The model under review builds one solid part; all positions refer to its coordinate system, in mm. Face numbers are marked on the shaded views. A direction names the side the tool comes from. Round coordinates to 2 decimals unless told otherwise and drop trailing zeros. Order: outer loops, then holes, each group sorted by start corner. A loop starts at its lowest first (then second) coordinate and runs counter-clockwise, first axis right, second up. Notation, with made-up numbers: M 85.25,-1 L 144.25,-1 A24 ccw 144.25,25 Z; hole C 32.5,52.25 d3. An arc over 180 degrees is marked long. Answer as a JSON object with one key per item and string values. Group by question number.
1) The part is to be moulded in two halves that separate along X. For the marked faces 1, 2 and 3, say which applies: +X half, -X half, draft (parallel to the pull), parting line (faces both ways), or undercut.
2) Consider section B-B, the plane y = 0.35. Write out the cut boundary in (x, z) (3 decimals), then the cut area to 3 significant figures.
3) Insertion check: pin 1 Ø1.3 at (x, z) = (-0.5, -0.5) entering from +Y; pin 2 Ø1 at (x, y) = (-10, 0.5) entering from -Z; pin 3 Ø2.5 at (x, z) = (0, 0) entering from -Y; pin 4 Ø1 at (x, y) = (1, 1.5) entering from -Z. Each pin has a flat end and moves straight along its axis. Give the tip position at first contact, or say it passes through.
4) Consider section C-C, the plane z = -0.25. Write out the cut boundary in (x, y).
5) Consider section D-D, the plane x = 2. Write out the cut boundary in (y, z).
6) To check wall thickness, follow line 1 (Y direction, x = -9.5, z = 0); line 2 (X direction, y = 3.25, z = 1.25); line 3 (Z direction, x = -0.75, y = 1.65). State the ranges of each line that lie inside material, in increasing order.
7) For the marked faces 4 and 5, list the 3-axis set-ups (+Z, -Z, +X, -X, +Y, -Y) from which the entire face can be reached by the end or side of a thin tool; tool diameter is ignored.
8) Consider section A-A, the plane x = 0. Write out the cut boundary in (y, z) (3 decimals), then the cut area to 3 significant figures.
```python
from build123d import *

# Parameters (mm, degrees)
ESTRUSIONE_ESTRUSIONE1_DEPTH = 1.35
SCHIZZO2_R                   = 3.375
ESTRUSIONE_ESTRUSIONE2_DEPTH = 2
SCHIZZO3_R                   = 2.25
TAGLIO_ESTRUSIONE1_DEPTH     = 2
SCHIZZO4_R                   = 1
TAGLIO_ESTRUSIONE2_DEPTH     = 17.47393775


with BuildPart() as part:
    # Schizzo1 → Estrusione-Estrusione1 (new body)
    with BuildSketch(Plane(origin=(0, 0, 0), x_dir=(1, 0, 0), z_dir=(0, 1, 0))):
        with BuildLine():
            ThreePointArc((-2.090005981, -2.65), (-3.375, 0), (-2.090005981, 2.65))
            Line((-2.090005981, 2.65), (-14.5, 1.5))
            ThreePointArc((-14.5, 1.5), (-16, 0), (-14.5, -1.5))
            Line((-14.5, -1.5), (-2.090005981, -2.65))
        make_face()
        with BuildLine():
            ThreePointArc((3.375, 0), (1.472558117, 3.036807138), (-2.090005981, 2.65))
            Line((-2.090005981, 2.65), (-2.090005981, -2.65))
            ThreePointArc((-2.090005981, -2.65), (1.472558117, -3.036807138), (3.375, 0))
        make_face()
        with BuildLine():
            Line((-2.090005981, -2.65), (-2.090005981, 2.65))
            ThreePointArc((-2.090005981, 2.65), (-3.375, 0), (-2.090005981, -2.65))
        make_face()
    extrude(amount=ESTRUSIONE_ESTRUSIONE1_DEPTH)

    # Schizzo2 → Estrusione-Estrusione2 (add)
    with BuildSketch(Plane(origin=(0, 1.35, 0), x_dir=(1, 0, 0), z_dir=(0, 1, 0))):
        with Locations(Location((0, 0, 0), (0, 0, 128.262191128))):
            Circle(SCHIZZO2_R)
    extrude(amount=ESTRUSIONE_ESTRUSIONE2_DEPTH)

    # Schizzo3 → Taglio-Estrusione1 (cut)
    with BuildSketch(Plane(origin=(0, 3.35, 0), x_dir=(1, 0, 0), z_dir=(0, 1, 0))):
        with Locations(Location((0, 0, 0), (0, 0, 270))):
            Circle(SCHIZZO3_R)
    extrude(amount=-TAGLIO_ESTRUSIONE1_DEPTH, mode=Mode.SUBTRACT)

    # Schizzo4 → Taglio-Estrusione2 (cut, through all)
    with BuildSketch(Plane(origin=(0, 1.35, 0), x_dir=(1, 0, 0), z_dir=(0, 1, 0))):
        with Locations(Location((0, 0, 0), (0, 0, 270))):
            Circle(SCHIZZO4_R)
    extrude(amount=-TAGLIO_ESTRUSIONE2_DEPTH, mode=Mode.SUBTRACT)


solid = part.part
```
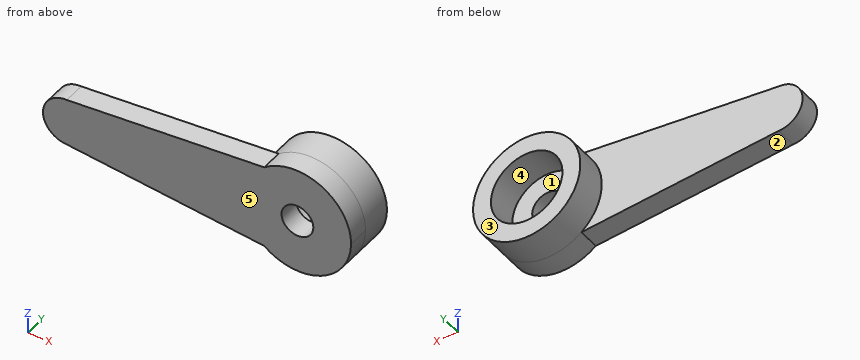
Results list:
{
 "1": {"face 1": "undercut", "face 2": "-X half", "face 3": "draft"},
 "2": {"outline": "M -14.5,-1.5 L -2.09,-2.65 A3.375 ccw long -2.09,2.65 L -14.5,1.5 A1.5 ccw Z; hole C 0,0 d2", "area": "82.9 mm^2"},
 "3": {"pin 1": "y = 1.35", "pin 2": "z = -1.96", "pin 3": "y = 0", "pin 4": "z = -3.34"},
 "4": {"outline": "M -15.98,0 L -0.97,0 L -0.97,1.35 L -2.24,1.35 L -2.24,3.35 L -3.37,3.35 L -3.37,1.35 L -15.98,1.35 Z; M 0.97,0 L 3.37,0 L 3.37,3.35 L 2.24,3.35 L 2.24,1.35 L 0.97,1.35 Z"},
 "5": {"outline": "M 0,-2.72 L 3.35,-2.72 L 3.35,-1.03 L 1.35,-1.03 L 1.35,1.03 L 3.35,1.03 L 3.35,2.72 L 0,2.72 Z"},
 "6": {"line 1": "0 to 1.35", "line 2": "-3.13 to -1.87, 1.87 to 3.13", "line 3": "-3.29 to -2.12, 2.12 to 3.29"},
 "7": {"face 4": "+Y", "face 5": "+Z, -Z, +X, -X, -Y"},
 "8": {"outline": "M 0,-3.375 L 3.35,-3.375 L 3.35,-2.25 L 1.35,-2.25 L 1.35,-1 L 0,-1 Z; M 0,1 L 1.35,1 L 1.35,2.25 L 3.35,2.25 L 3.35,3.375 L 0,3.375 Z", "area": "10.9 mm^2"}
}
